```python
from build123d import *

# Parameters (mm, degrees)
SKETCH1_W                = 78.486
SKETCH1_H                = 113.03
BOSS_EXTRUDE1_DEPTH      = 68.326
BOSS_EXTRUDE1_DEPTH_BACK = 15.494
SHELL1_T                 = -17.78
SHELL5_T                 = -2.54
SKETCH2_W                = 50.166140906
SKETCH2_H                = 33.974952571
CUT_EXTRUDE1_DEPTH       = 12.446
F_0_80_TAPPED_HOLE1_D    = 1.19126


with BuildPart() as part:
    # Sketch1 → Boss-Extrude1 (new body, two sides)
    with BuildSketch(Plane(origin=(0, 0, 0), x_dir=(1, 0, 0), z_dir=(0, 1, 0))) as boss_extrude1_sk:
        Rectangle(SKETCH1_W, SKETCH1_H)
    extrude(amount=BOSS_EXTRUDE1_DEPTH)
    extrude(boss_extrude1_sk.sketch, amount=-BOSS_EXTRUDE1_DEPTH_BACK)

    # Shell1
    shell1_openings = [part.faces().sort_by_distance(p)[0] for p in [
        (0, 68.326, 0),
    ]]
    offset(amount=SHELL1_T, openings=shell1_openings, kind=Kind.INTERSECTION)

    # Shell5
    shell5_openings = [part.faces().sort_by_distance(p)[0] for p in [
        (39.243, 26.416, 0),
    ]]
    offset(amount=SHELL5_T, openings=shell5_openings, kind=Kind.INTERSECTION)

    # Sketch2 → Cut-Extrude1 (cut)
    with BuildSketch(Plane(origin=(24.003, 0, 0), x_dir=(0, 0, -1), z_dir=(1, 0, 0))):
        with Locations((0, 38.426676593)):
            Rectangle(SKETCH2_W, SKETCH2_H)
    extrude(amount=-CUT_EXTRUDE1_DEPTH, mode=Mode.SUBTRACT)

    # #0-80 Tapped Hole1 (through all)
    with Locations(Plane(origin=(0, 68.326, 0), x_dir=(1, 0, 0), z_dir=(0, 1, 0))):
        with Locations((-31.94519897, 51.782137041), (-32.97568926, 45.942692068), (28.853728102, 51.782137041), (31.258205444, 45.942692068), (31.258205444, -46.114440449), (28.853728102, -50.236401607), (-31.94519897, -50.236401607), (-32.97568926, -43.194717963)):
            Hole(F_0_80_TAPPED_HOLE1_D / 2)


solid = part.part
```
Geometry check sheet. Reference: the model listing, model coordinates, mm. A direction names the side the tool comes from. Round coordinates to 2 decimals unless told otherwise and drop trailing zeros. Loops run counter-clockwise (first coordinate to the right, second up) from the corner with the lowest first, then second, coordinate; pieces in that order, holes last. Notation, with made-up numbers: (10.25, -0.5) -> (37.25, -0.5) arc R15 ccw to (37.25, 23.5) -> close; hole circle Ø6 at (-36, -37). An arc over 180 degrees is marked (long way). Use a Markdown table: item, result.
(1) Sectioned sample at B-B (z = 19). Enter the section's corners in (x, y).
Calculated:
| item | result |
|---|---|
| outline | (-39.24, -15.49) -> (39.24, -15.49) -> (39.24, -12.95) -> (-36.7, -12.95) -> (-36.7, 65.79) -> (-24, 65.79) -> (-24, -0.25) -> (24, -0.25) -> (24, 21.44) -> (21.46, 21.44) -> (21.46, 2.29) -> (-21.46, 2.29) -> (-21.46, 68.33) -> (-39.24, 68.33) -> close; (21.46, 55.41) -> (24, 55.41) -> (24, 65.79) -> (39.24, 65.79) -> (39.24, 68.33) -> (21.46, 68.33) -> close |
(2) Sectioned sample at C-C (y = 28.5). Enter the section's corners in (x, z) (3 decimals), then the cut area to 3 significant figures.
Calculated:
| item | result |
|---|---|
| outline | (-39.243, -56.515) -> (39.243, -56.515) -> (39.243, -53.975) -> (-36.703, -53.975) -> (-36.703, 53.975) -> (39.243, 53.975) -> (39.243, 56.515) -> (-39.243, 56.515) -> close; (-24.003, -41.275) -> (24.003, -41.275) -> (24.003, -25.083) -> (21.463, -25.083) -> (21.463, -38.735) -> (-21.463, -38.735) -> (-21.463, 38.735) -> (21.463, 38.735) -> (21.463, 25.083) -> (24.003, 25.083) -> (24.003, 41.275) -> (-24.003, 41.275) -> close |
| area | 1,180 mm² |
(3) Sectioned sample at A-A (y = 7). Enter the section's corners in (x, z) (3 decimals).
Calculated:
| item | result |
|---|---|
| outline | (-39.243, -56.515) -> (39.243, -56.515) -> (39.243, -53.975) -> (-36.703, -53.975) -> (-36.703, 53.975) -> (39.243, 53.975) -> (39.243, 56.515) -> (-39.243, 56.515) -> close; (-24.003, -41.275) -> (24.003, -41.275) -> (24.003, 41.275) -> (-24.003, 41.275) -> close; hole (-21.463, -38.735) -> (21.463, -38.735) -> (21.463, 38.735) -> (-21.463, 38.735) -> close |
(4) Go/stop test with flat-tipped pins: P1, Ø1.5, axis at x = 28.85, z = 50.24, coming from the +Y side; P2, Ø6, axis at y = 27.5, z = 41, coming from the +X side; P3, Ø13, axis at x = 7, z = -14.5, coming from the +Y side. Record where each tip stops, or that it passes through.
Calculated:
| item | result |
|---|---|
| P1 | y = 68.33 |
| P2 | x = 24 |
| P3 | y = 2.29 |
(5) Mould release check, pull along X, two halves, no side actions. Record for faces 1 (the flat face through (0, 33, -41.275)), 2 (the flat face through (21.463, 21, 1)), 3 (the flat face through (24.003, 19, 1)): released by +X, released by -X, zero draft, split by the parting line, or undercut.
Calculated:
| item | result |
|---|---|
| face 1 | zero draft |
| face 2 | undercut |
| face 3 | released by +X |
(6) Sectioned sample at D-D (x = 1.5). Enter the section's corners in (y, z) (3 decimals).
Calculated:
| item | result |
|---|---|
| outline | (-15.494, -56.515) -> (68.326, -56.515) -> (68.326, -38.735) -> (2.286, -38.735) -> (2.286, 38.735) -> (68.326, 38.735) -> (68.326, 56.515) -> (-15.494, 56.515) -> close; hole (-12.954, -53.975) -> (65.786, -53.975) -> (65.786, -41.275) -> (-0.254, -41.275) -> (-0.254, 41.275) -> (65.786, 41.275) -> (65.786, 53.975) -> (-12.954, 53.975) -> close |
(7) Set-up check for faces 4 (the flat face through (-1, 27, -56.515)), 5 (the flat face through (0, 36, -38.735)), 6 (the flat face through (-36.703, 27, 1)), 7 (the flat face through (1, 27, -53.975)), 8 (the flat face through (-27, 68.326, -1)): record each of +Z, -Z, +X, -X, +Y, -Y from which the full face is reachable in a straight line by a thin tool's end or side.
Calculated:
| item | result |
|---|---|
| face 4 | -Z, +X, -X, +Y, -Y |
| face 5 | +Y |
| face 6 | none |
| face 7 | +X |
| face 8 | +Z, -Z, +X, -X, +Y |
(8) Scan lines: probe 1 along Z at (x, y) = (11.5, 20) (3 decimals); probe 2 along Z at (x, y) = (21.5, 48) (3 decimals); probe 3 along X at (y, z) = (35.5, -36). Record each from-to range of solid material in increasing order.
Calculated:
| item | result |
|---|---|
| probe 1 | -56.515 to -53.975, -41.275 to -38.735, 38.735 to 41.275, 53.975 to 56.515 |
| probe 2 | -56.515 to -53.975, -41.275 to -25.083, 25.083 to 41.275, 53.975 to 56.515 |
| probe 3 | -39.24 to -36.7, -24 to -21.46, 21.46 to 24 |
